Autodesk Inventor part; units mm, degrees
ref_plane "WorkPlane1" through (0, 0, 0) normal (0, 0, 1) x (1, 0, 0)
ref_plane "Work Plane2" through (0, 0, -1.2) normal (0, 0, 1) x (1, 0, 0)
ref_plane "WorkPlane2" through (0, 0, 1.5) normal (0, 0, 1) x (1, 0, 0)
ref_plane "WorkPlane1" through (0, 0, 0) normal (0, 0, 1) x (1, 0, 0)
ref_plane "Work Plane2" through (0, 0, -1.2) normal (0, 0, 1) x (1, 0, 0)
ref_plane "WorkPlane2" through (0, 0, 1.5) normal (0, 0, 1) x (1, 0, 0)
sketch "Boceto1" plane through (0, 0, 0) normal (0, 0, 1) x (1, 0, 0)
  point P0 (0, 0)
sketch "Boceto2" plane through (0, 0, 0) normal (0, 0, 1) x (1, 0, 0)
  line L0 (5, -13.947) -> (5, -10.8655)
  line L1 (1, -14.6523) -> (5, -13.947)
  line L2 (1, -10.4523) -> (1, -14.6523)
  arc A0 (1, -10.4523) -> (-1, -10.4523) centre (0, 0) ccw
  line L3 (-1, -10.4523) -> (-1, -14.6523)
  line L4 (-1, -14.6523) -> (-5, -13.947)
  line L5 (-5, -13.947) -> (-5, -10.8655)
  arc A1 (5, -10.8655) -> (-5, -10.8655) centre (0, 0.7) ccw
  dimension "d2" = 10.5
  dimension "d4" = 12.6
  dimension "d6" = 0
  dimension "d8" = 1
  dimension "d10" = 1
  dimension "d12" = 4.2
  dimension "d14" = 4.2
  dimension "d16" = 80
  dimension "d18" = 80
  dimension "d20" = 4
  dimension "d22" = 4
  dimension "d24" = 0.7
  dimension "d52" = 0
  dimension "d53" = 0
extrude "Extrusión1" add sketch "Boceto2" along normal blind 1.2
sketch "Boceto3" plane through (0, 0, 1.2) normal (0, 0, 1) x (1, 0, 0)
  line L0 (-1, -10.4523) -> (-1, -14.6523)
  line L1 (-1, -14.6523) -> (-5, -13.947)
  point P0 (-2.6, -12.451)
  dimension "d30" = 1.6
  dimension "d32" = 1.89
hole "Agujero1" at (-2.6, -12.451, 1.2) direction (0, 0, -1) diameter 2 end through all
sketch "Boceto4" plane through (0, 0, 1.2) normal (0, 0, 1) x (1, 0, 0)
  line L0 (1, -14.6523) -> (1, -10.4523)
  line L1 (5, -13.947) -> (1, -14.6523)
  point P0 (2.6, -12.451)
  dimension "d41" = 1.6
  dimension "d43" = 1.89
hole "Agujero2" at (2.6, -12.451, 1.2) direction (0, 0, -1) diameter 2 end through all
fillet "Empalme1" radius 3 2 edges at (-5, -13.947, 0.6) (5, -13.947, 0.6)
equation "\"d2\" = 0.5 * Diam2"
equation "\"d4\" = 0.166667 * ParA + 0.5 * Diam2 + 0.5 * b"
equation "\"d8\" = 0.5 * Diam5"
equation "\"d10\" = 0.5 * Diam5"
equation "\"d12\" = ParA"
equation "\"d14\" = ParA"
equation "\"d20\" = 2 * Diam5"
equation "\"d22\" = 2 * Diam5"
equation "\"d24\" = -msp_r2 + 0.5 * Diam2 + b"
equation "\"d25\" = ParS"
equation "\"d33\" = Diam5"
equation "\"d44\" = Diam5"
equation "\"d51\" = 1.5 * Diam5"
equation "\"Diam5\" = 2"
equation "\"ParA\" = 4.2"
equation "\"ParS\" = 1.2"
equation "\"Diam2\" = 21"
equation "\"msp_r2\" = 0.166667 * ParA + 0.5 * Diam2 + 0.5 * b"
equation "\"TEMPLATE\" = 1.2345"
properties part number "DIN 471 - 22x1,2" material "Acero, suave"
Can you work these out from the model? Positions are in its coordinate system, mm. A direction names the side the tool comes from. Coordinates: 2 decimals unless noted, no trailing zeros. Write each loop counter-clockwise with the first axis right and the second up, starting at its lowest first coordinate (ties: lowest second). Pieces come first, ordered by that corner, then holes. Notation, with made-up numbers: M 21.25,-40 L 78.25,-40 A19 cw 78.25,-21 Z; hole C 49.5,-36.75 d2. An arc over 180 degrees is marked long. Answer as CSV lines item,"result".
Item 1: Imagine slicing it at A-A on z = 0.5. List the corners of the cut face in (x, y) for me, plus the area to 3 significant figures.
Geometry results:
outline,"M -5,-11.43 A3 ccw -2.52,-14.38 L -1,-14.65 L -1,-10.45 A10.5 cw long 1,-10.45 L 1,-14.65 L 2.52,-14.38 A3 ccw 5,-11.43 L 5,-10.87 A12.6 ccw long -5,-10.87 Z; hole C -2.6,-12.45 d2; hole C 2.6,-12.45 d2"
area,"163 mm2"
Item 2: We'd pull the mould along Y, two halves only. Please class faces 3 (the cylindrical face through (-0.45, 10.49, 0.59)), 4 (the cylindrical face through (-0.48, 13.29, 0.59)), 5 (the flat face through (-1, 11, 0)), 6 (the cylindrical face through (-4.317, -13.336, 0.608)): +Y half, -Y half, draft (parallel to the pull), parting line (faces both ways), or undercut.
Geometry results:
face 3,"undercut"
face 4,"parting line"
face 5,"draft"
face 6,"-Y half"
Item 3: Imagine slicing it at C-C on x = -9. List the corners of the cut face in (y, z) for me, plus the area to 3 significant figures.
Geometry results:
outline,"M -8.12,0 L -5.41,0 L -5.41,1.2 L -8.12,1.2 Z; M 5.41,0 L 9.52,0 L 9.52,1.2 L 5.41,1.2 Z"
area,"8.18 mm2"
Item 4: Please list where these lines run through material, in increasing order: line 1 along Y through (x, z) = (2.6, 0.7); line 2 along Y through (x, z) = (0, 0.35); line 3 along X through (y, z) = (-11.25, 0.15).
Geometry results:
line 1,"y = -14.37 to -13.45, -11.45 to -10.17, 10.17 to 13.03"
line 2,"y = 10.5 to 13.3"
line 3,"x = -5 to -1, 1 to 5"
Item 5: On a 3-axis mill with a long thin cutter (end or side, diameter ignored), from which of +Z, -Z, +X, -X, +Y, -Y can I reach the whole of each face in a straight line? I mean faces 1 (the cylindrical face through (4.28, -13.38, 0.61)), 2 (the flat face through (1, -13, 1)). Say none if no direction works.
Geometry results:
face 1,"+Z, -Z, +X, -Y"
face 2,"+Z, -Z, -Y"
Item 6: I'm going to push flat-ended pins straight in: P1, Ø0.6, axis at y = -11, z = 0.5, coming from the -X side; P2, Ø0.6, axis at y = -12.5, z = 0.5, coming from the -X side; P3, Ø12.5, axis at x = 0, y = 0, coming from the +Z side; P4, Ø0.5, axis at y = -11, z = 0.5, coming from the +X side. Where does each tip first touch, or does it pass through?
Geometry results:
P1,"stops at x = -5.37"
P2,"stops at x = -4.9"
P3,"passes through"
P4,"stops at x = 5.26"
Item 7: Imagine slicing it at B-B on y = 0. List the corners of the cut face in (x, z) for me.
Geometry results:
outline,"M -12.58,0 L -10.5,0 L -10.5,1.2 L -12.58,1.2 Z; M 10.5,0 L 12.58,0 L 12.58,1.2 L 10.5,1.2 Z"
Item 8: Imagine slicing it at D-D on x = -3. List the corners of the cut face in (y, z) for me, plus the area to 3 significant figures.
Geometry results:
outline,"M -14.26,0 L -13.37,0 L -13.37,1.2 L -14.26,1.2 Z; M -11.53,0 L -10.06,0 L -10.06,1.2 L -11.53,1.2 Z; M 10.06,0 L 12.94,0 L 12.94,1.2 L 10.06,1.2 Z"
area,"6.29 mm2"
